Verification items for the finished model (mm, model axes). A direction names the side the tool comes from. Give positions to 0.01 mm unless a question says otherwise; leave off trailing zeros. Use a Markdown table: item, result.
from build123d import *

# Parameters (mm, degrees)
F1_W      = 24.9
F1_H      = 16.1
F2_W      = 18.339114
F2_H      = 15.596803
F4_W      = 9.09091
F4_H      = 28
F5_DEPTH  = 43.97606
F7_DEPTH  = 48.58648
F8_R      = 1.628979
F9_DEPTH  = 25
F10_R     = 1.57945
F11_DEPTH = 25


with BuildPart() as f3:
    # F1 (on Top) → F3 section 0
    with BuildSketch(Plane.XY):
        with Locations((-36.237153, 30.487152)):
            Rectangle(F1_W, F1_H)
    # F2 (on offset) → F3 section 1
    with BuildSketch(Plane.XY.offset(40)):
        with Locations((-32.853606, 30.5409)):
            Rectangle(F2_W, F2_H)
    loft()

    # F4 (on Front) → F5 (cut)
    with BuildSketch(Plane.XZ):
        with Locations((-33.169536, 19.06869)):
            Rectangle(F4_W, F4_H)
    extrude(amount=-F5_DEPTH, mode=Mode.SUBTRACT)

    # F6 (on Right) → F7 (cut)
    with BuildSketch(Plane.YZ):
        with BuildLine():
            ThreePointArc((33.29777, 25.870029), (29.562821, 29.604978), (25.827872, 25.870029))
            Line((25.827872, 25.870029), (25.827872, 15.214866))
            ThreePointArc((25.827872, 15.214866), (29.562821, 11.479917), (33.29777, 15.214866))
            Line((33.29777, 15.214866), (33.29777, 25.870029))
        make_face()
    extrude(amount=-F7_DEPTH, mode=Mode.SUBTRACT)

    # F8 (on offset) → F9 (cut)
    with BuildSketch(Plane.XY.offset(40)):
        with Locations((-32.914963, 33.718325)):
            Circle(F8_R)
    extrude(amount=-F9_DEPTH, mode=Mode.SUBTRACT)

    # F10 (on offset) → F11 (cut)
    with BuildSketch(Plane.XY.offset(40)):
        with Locations((-32.921717, 28.86181)):
            Circle(F10_R)
    extrude(amount=-F11_DEPTH, mode=Mode.SUBTRACT)


solid = f3.part
(1) Gauge pin test, flat ends, axial feed: P1, Ø4, axis at x = -41, z = 19, coming from the -Y side; P2, Ø6, axis at y = 36, z = 34.5, coming from the +X side; P3, Ø5, axis at y = 29.5, z = 10, coming from the -X side; P4, Ø3.5, axis at x = -32.92, y = 28.86, coming from the +Z side. Record the tip position at first contact, or that the pin passes through.
Results below:
| item | result |
|---|---|
| P1 | y = 22.57 |
| P2 | x = -23.69 |
| P3 | x = -47.44 |
| P4 | z = 40 |
(2) Cross-section at A-A on x = -33.5. State how many separate pieces and enclosed holes the cut face has, then the cut area to 3 significant figures.
Results below:
| item | result |
|---|---|
| separate pieces | 4 |
| enclosed holes | 0 |
| area | 148 mm^2 |
(3) Draft check along X on faces 4 (the flat face through (-26, 33.298, 20)), 5 (the flat face through (-33, 30, 5.069)), 6 (the cylindrical face through (-33.127, 35.333, 36.583)). Enter one of: +X half, -X half, draft (parallel to the pull), parting line (faces both ways), or undercut.
Results below:
| item | result |
|---|---|
| face 4 | draft |
| face 5 | undercut |
| face 6 | undercut |
(4) Material ranges on line 1 (Z direction, x = -35.5, y = 29.5); line 2 (X direction, y = 25, z = 16) (3 decimals); line 3 (X direction, y = 24.25, z = 31) (3 decimals), recorded low to high.
Results below:
| item | result |
|---|---|
| line 1 | 0 to 5.07, 33.07 to 40 |
| line 2 | -46.022 to -37.715, -28.624 to -23.746 |
| line 3 | -43.523 to -37.715, -28.624 to -23.707 |
(5) Set-up check for faces 1 (the cylindrical face through (-32.19, 27.46, 36.58)), 2 (the flat face through (-34.2, 30.4, 33.069)), 3 (the flat face through (-42, 25.828, 21)): record each of +Z, -Z, +X, -X, +Y, -Y from which the full face is reachable in a straight line by a thin tool's end or side.
Results below:
| item | result |
|---|---|
| face 1 | +Z |
| face 2 | +Y, -Y |
| face 3 | +X, -X |
